The model under review builds one solid part; all positions refer to its coordinate system, in mm. Face numbers are marked on the shaded views. Give positions to 0.01 mm unless a question says otherwise; leave off trailing zeros. Order: outer loops, then holes, each group sorted by start corner. A loop starts at its lowest first (then second) coordinate and runs counter-clockwise, first axis right, second up. Notation, with made-up numbers: (46, -16) -> (57, -16) arc R37 cw to (57, 20) -> close; hole circle Ø6 at (54, 1). An arc over 180 degrees is marked (long way). Use one line per item in the form item = value.
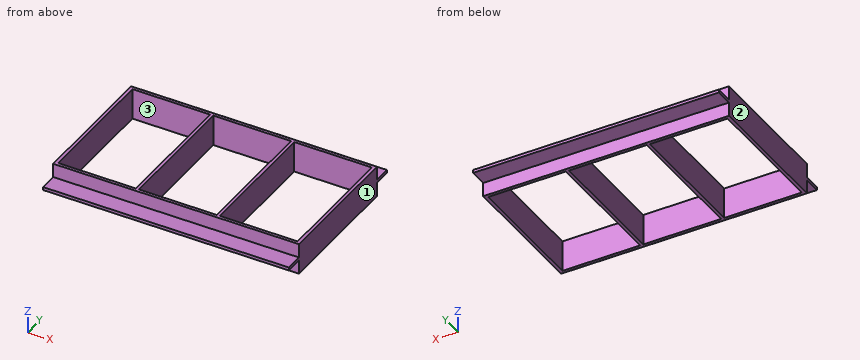
```python
from build123d import *

# Parameters (mm, degrees)
F0_W     = 948
F0_H     = 524
F0_W_2   = 300
F0_H_2   = 500
F1_DEPTH = 120
F3_DEPTH = 948


with BuildPart() as f1:
    # F0 (on Top) → F1 (new body)
    with BuildSketch(Plane.XY):
        Rectangle(F0_W, F0_H)
        with Locations((-312, 0)):
            Rectangle(F0_W_2, F0_H_2, mode=Mode.SUBTRACT)
        Rectangle(F0_W_2, F0_H_2, mode=Mode.SUBTRACT)
        with Locations((312, 0)):
            Rectangle(F0_W_2, F0_H_2, mode=Mode.SUBTRACT)
    extrude(amount=F1_DEPTH)

    # F2 (on face) → F3 (join, through all)
    with BuildSketch(Plane(origin=(-474, 0, 0), x_dir=(0, -1, 0), z_dir=(-1, 0, 0))):
        Polygon((-330, 54), (-262, 54), (-262, 66), (-330, 66), (-330, 60), align=None)
        Polygon((262, 66), (262, 54), (330, 54), (330, 60), (330, 66), align=None)
    extrude(amount=-F3_DEPTH)


solid = f1.part
```
1. Add section B-B on y = -108. Give the boundary of the cut face in (x, z), then the cut area to 3 significant figures.
Values:
outline = (-474, 0) -> (-462, 0) -> (-462, 120) -> (-474, 120) -> close; (-162, 0) -> (-150, 0) -> (-150, 120) -> (-162, 120) -> close; (150, 0) -> (162, 0) -> (162, 120) -> (150, 120) -> close; (462, 0) -> (474, 0) -> (474, 120) -> (462, 120) -> close
area = 5,760 mm^2
2. Add section A-A on z = 91.5. Give the boundary of the cut face in (x, y).
Values:
outline = (-474, -262) -> (474, -262) -> (474, 262) -> (-474, 262) -> close; hole (-462, -250) -> (-162, -250) -> (-162, 250) -> (-462, 250) -> close; hole (-150, -250) -> (150, -250) -> (150, 250) -> (-150, 250) -> close; hole (162, -250) -> (462, -250) -> (462, 250) -> (162, 250) -> close
3. Add section D-D on y = -289.5. Give the boundary of the cut face in (x, z).
Values:
outline = (-474, 54) -> (474, 54) -> (474, 66) -> (-474, 66) -> close
4. For pin 1 Ø1 at (x, z) = (-242, 20.5) entering from -Y; pin 2 Ø16 at (x, z) = (-123, 85.5) entering from +Y; pin 3 Ø20.5 at (x, y) = (48.5, 310.5) entering from +Z; pin 4 Ø3 at (x, z) = (92, 53.5) entering from +Y, all flat-tipped, find the tip position at first contact; note any pin that passes through.
Values:
pin_1 = -262
pin_2 = 262
pin_3 = 66
pin_4 = 330
5. For L1, parallel to X at y = 107, z = 12; L2, parallel to Y at x = -49.5, z = 94.5; L3, parallel to Y at x = 120, z = 62.5, list the stretches that pass through material, from the lowest coordinate up.
Values:
L1 = -474 to -462, -162 to -150, 150 to 162, 462 to 474
L2 = -262 to -250, 250 to 262
L3 = -330 to -250, 250 to 330
6. Add section C-C on x = -361. Give the boundary of the cut face in (y, z), then the cut area to 3 significant figures.
Values:
outline = (-330, 54) -> (-262, 54) -> (-262, 0) -> (-250, 0) -> (-250, 120) -> (-262, 120) -> (-262, 66) -> (-330, 66) -> close; (250, 0) -> (262, 0) -> (262, 54) -> (330, 54) -> (330, 66) -> (262, 66) -> (262, 120) -> (250, 120) -> close
area = 4,510 mm^2
7. The part is to be moulded in two halves that separate along X. For the marked faces 1, 2 and 3, say which applies: +X half, -X half, draft (parallel to the pull), parting line (faces both ways), or undercut.
Values:
face_1 = +X half
face_2 = -X half
face_3 = undercut
